Geometry check sheet. Reference: drawing and pictorial views, mm from the part's lowest x, y, z. Round coordinates to 2 decimals unless told otherwise and drop trailing zeros. Write each loop counter-clockwise with the first axis right and the second up, starting at its lowest first coordinate (ties: lowest second). Pieces come first, ordered by that corner, then holes. Notation, with made-up numbers: M -17,56 L 6,56 A27 ccw 6,75 Z; hole C 48,41.25 d2. An arc over 180 degrees is marked long. Put each result on its own line as item: value. Start each with the question number.
(1) Material ranges on probe 1 along Y at (x, z) = (46.5, 2.05); probe 2 along X at (y, z) = (53, 0.65); probe 3 along X at (y, z) = (65.5, 2.6), recorded low to high.
(2) Section check A-A on y = 78.5. Record the cut outline in (x, z).
(3) Section check D-D on y = 18.5. Record the cut outline in (x, z), then the cut area to 3 significant figures.
(4) Section check B-B on x = 227. Record the cut outline in (y, z).
(5) Section check C-C on z = 2.8. Record the cut outline in (x, y).
(6) Gauge pin test, flat ends, axial feed: pin 1 (2 mm diameter, centred on y = 100, z = 2, fed in from +X); pin 2 (1.5 mm diameter, centred on x = 279.5, z = 3.5, fed in from -Y) (1 decimal). Record the tip position at first contact, or that the pin passes through.
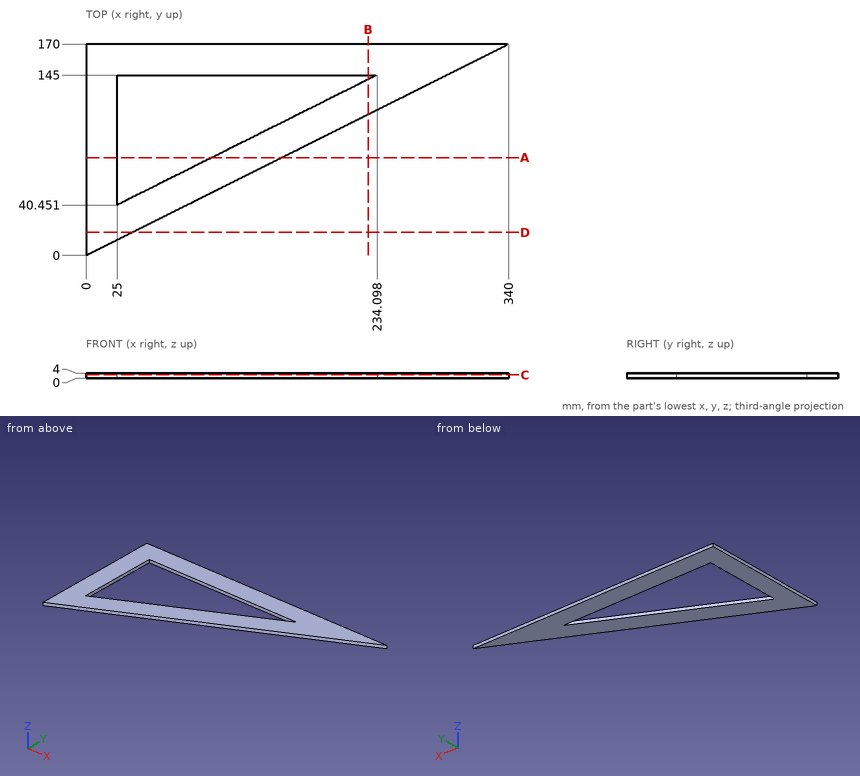
Answers follow:
1. probe 1: y = 23.25 to 51.2, 145 to 170
1. probe 2: x = 0 to 25, 50.1 to 106
1. probe 3: x = 0 to 25, 75.1 to 131
2. outline: M 0,0 L 25,0 L 25,4 L 0,4 Z; M 101.1,0 L 157,0 L 157,4 L 101.1,4 Z
3. outline: M 0,0 L 37,0 L 37,4 L 0,4 Z
3. area: 148 mm^2
4. outline: M 113.5,0 L 141.45,0 L 141.45,4 L 113.5,4 Z; M 145,0 L 170,0 L 170,4 L 145,4 Z
5. outline: M 0,0 L 340,170 L 0,170 Z; hole M 25,40.45 L 234.1,145 L 25,145 Z
6. pin 1: stops at x = 202
6. pin 2: stops at y = 139.4
